Could you check a few things on this model? Use its own coordinates, in mm. Face numbers are marked on the shaded views. Coordinates: 2 decimals unless noted, no trailing zeros. Loops run counter-clockwise (first coordinate to the right, second up) from the corner with the lowest first, then second, coordinate; pieces in that order, holes last. Notation, with made-up numbers: (50.25, 41) -> (100.25, 41) arc R14 ccw to (100.25, 62) -> close; hole circle Ø11 at (13.5, 71.5). An arc over 180 degrees is marked (long way). One line per question, with ' | ' between items. Start each with the question number.
(1) Suppose I cut it at C-C (x = 36.5). Please give me the cut outline in (y, z).
(2) If I drill on line 1 along Y through (x, z) = (4, 0); line 2 along Y through (x, z) = (43, 23), over which ranges is the centre line in solid material (lowest first)?
(3) I'm going to push flat-ended pins straight in: pin 1 Ø4 at (x, y) = (4.5, -15) entering from +Z; pin 2 Ø1.5 at (x, z) = (-6.5, 24.5) entering from -Y; pin 3 Ø10 at (x, z) = (-44.5, -33.5) entering from -Y. Where does each tip first touch, or does it pass through?
(4) Suppose I cut it at B-B (z = -27). Please give me the cut outline in (x, y), plus the area to 3 significant figures.
(5) Suppose I cut it at D-D (y = 40). Please give me the cut outline in (x, z).
(6) If we mould it in two halves opening along Y, with no side actions, what happens to the marked faces 1, 2 and 3? For each: pulls with the +Y half, pulls with the -Y half, needs draft (parallel to the pull), parting line crosses it, or undercut.
(7) Suppose I cut it at A-A (y = 0). Please give me the cut outline in (x, z).
```python
from build123d import *

# Parameters (mm, degrees)
F0_W     = 160
F0_H     = 14
F3_DEPTH = 45.8700225313


# Not quite as in the source:
# - the program builds the solid bodies; features that only make, move or delete a surface that nothing else refers to are left out


with BuildPart() as f1:
    # F0 (on Front) → F1 (revolve)
    with BuildSketch(Plane.XZ):
        with Locations((0.4038456827, 38.8690225313)):
            Rectangle(F0_W, F0_H)
    revolve(axis=Axis((59.6884675324, 0, 0), (1, 0, 0)))

    # F2 (on Front) → F3 (cut, through all)
    with BuildSketch(Plane.XZ):
        with BuildLine():
            ThreePointArc((-38.8187138988, 0), (-40.2831799929, 3.5355339059), (-43.8187138988, 5))
            Line((-43.8187138988, 5), (-43.8187138988, -5))
            ThreePointArc((-43.8187138988, -5), (-40.2831799929, -3.5355339059), (-38.8187138988, 0))
        make_face()
        with BuildLine():
            Line((-43.8187138988, -5), (-43.8187138988, 5))
            ThreePointArc((-43.8187138988, 5), (-48.8187138988, 0), (-43.8187138988, -5))
        make_face()
    f3 = extrude(amount=F3_DEPTH, mode=Mode.SUBTRACT)

    # F4: F3 across plane
    add(f3.mirror(Plane.YZ), mode=Mode.SUBTRACT)


solid = f1.part
```
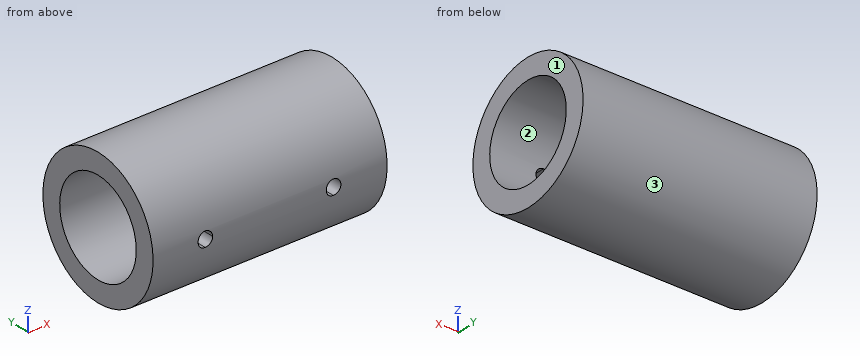
Checks:
1) outline: circle Ø91.74 at (0, 0); hole circle Ø63.74 at (0, 0)
2) line 1: y = -45.87 to -31.87, 31.87 to 45.87 | line 2: y = -39.69 to -22.06, 22.06 to 39.69
3) pin 1: stops at z = 43.99 | pin 2: stops at y = -39.24 | pin 3: stops at y = -35.94
4) outline: (-79.6, -37.08) -> (80.4, -37.08) -> (80.4, -16.93) -> (-79.6, -16.93) -> close; (-79.6, 16.93) -> (80.4, 16.93) -> (80.4, 37.08) -> (-79.6, 37.08) -> close | area: 6,450 mm^2
5) outline: (-79.6, -22.45) -> (80.4, -22.45) -> (80.4, 22.45) -> (-79.6, 22.45) -> close
6) face 1: needs draft | face 2: undercut | face 3: parting line crosses it
7) outline: (-79.6, -45.87) -> (80.4, -45.87) -> (80.4, -31.87) -> (-79.6, -31.87) -> close; (-79.6, 31.87) -> (80.4, 31.87) -> (80.4, 45.87) -> (-79.6, 45.87) -> close
